```python
from build123d import *

# Parameters (mm, degrees)
EXTRUDE_1_DEPTH          = 6
PATTERN_CIRCULAR_1_COUNT = 20
SKETCH_2_R               = 2.55
CUT_EXTRUDE_1_DEPTH      = 19


with BuildPart() as part:
    # 스케치1 → 보스-돌출1 (new body)
    with BuildSketch(Plane(origin=(0, 0, 0), x_dir=(0, 0, -1), z_dir=(1, 0, 0))):
        with BuildLine():
            ThreePointArc((0, 12), (1.10558919, 10.60769458), (1.5, 8.874119675))
            ThreePointArc((1.5, 8.874119675), (0, -9), (-1.5, 8.874119675))
            ThreePointArc((-1.5, 8.874119675), (-1.10558919, 10.60769458), (0, 12))
        make_face()
    extrude_1 = extrude(amount=EXTRUDE_1_DEPTH)

    # 원형 패턴1: 보스-돌출1 ×20 about axis
    pattern_circular_1_axis = Axis((0, 0, 0), (1, 0, 0))
    for i in range(1, PATTERN_CIRCULAR_1_COUNT):
        add(extrude_1.rotate(pattern_circular_1_axis, i * 360 / PATTERN_CIRCULAR_1_COUNT))

    # 스케치2 → 컷-돌출1 (cut, through all)
    with BuildSketch(Plane(origin=(6, 0, 0), x_dir=(0, 0, -1), z_dir=(1, 0, 0))):
        Circle(SKETCH_2_R)
    extrude(amount=-CUT_EXTRUDE_1_DEPTH, mode=Mode.SUBTRACT)


solid = part.part
```
The listing builds one solid part. Answer for the finished solid, in the listing's coordinates (mm). Coordinates: 2 decimals unless noted, no trailing zeros. Write each loop counter-clockwise with the first axis right and the second up, starting at its lowest first coordinate (ties: lowest second). Pieces come first, ordered by that corner, then holes. Notation, with made-up numbers: M -35.75,25 L 6.25,25 A11 ccw 6.25,35 Z; hole C 34.25,-29.75 d8. An arc over 180 degrees is marked long. Use a Markdown table: item, result. Add a question column.
1. Straight lines are drawn through the part: line 1 along Z through (x, y) = (2.2, 10.75); line 2 along Y through (x, z) = (2.2, -1); line 3 along Y through (x, z) = (3.4, -9.75). For each, find the intervals that lie inside material, in ascending order. Write a range as [from, to].
2. Given P1, Ø10, axis at y = -5, z = -6, coming from the -X side; P2, Ø2, axis at x = 4, z = -6.5, coming from the +Y side; P3, Ø1.5, axis at x = 5, z = 5.5, coming from the +Y side; P4, Ø1.5, axis at x = 2.5, y = -0.5, coming from the -Z side, each flat-ended and moving along its own axis, determine where each tip first touches the part or whether it passes through.
3. For a pull along Y with two mould halves and no side action, classify faces 1 (the cylindrical face through (2.958, 5.518, 9.322)), 2 (the cylindrical face through (2.96, 7.16, -8.13)) as +Y half, -Y half, draft (parallel to the pull), parting line (faces both ways), or undercut.
4. Section B-B (y = -10) is taken. Give the vertices of the cut face in (x, z).
5. Section D-D (z = -6) is taken. Give the vertices of the cut face in (x, y).
6. Section A-A (z = -2) is taken. Give the vertices of the cut face in (x, y), plus the area to 3 significant figures.
7. Section C-C (z = 8) is taken. Give the vertices of the cut face in (x, y).
Data:
| question | item | result |
|---|---|---|
| 1 | line 1 | z = [-4.06, -2.57], [-1.03, 1.03], [2.57, 4.06] |
| 1 | line 2 | y = [-10.81, -2.35], [2.35, 10.81] |
| 1 | line 3 | y = [-4.33, -1.7], [-1.4, 1.4], [1.7, 4.33] |
| 2 | P1 | stops at x = 0 |
| 2 | P2 | stops at y = 9.71 |
| 2 | P3 | stops at y = 9.59 |
| 2 | P4 | stops at z = -12 |
| 3 | face 1 | undercut |
| 3 | face 2 | undercut |
| 4 | outline | M 0,-4.29 L 6,-4.29 L 6,-1.87 L 0,-1.87 Z; M 0,-1.34 L 6,-1.34 L 6,1.34 L 0,1.34 Z; M 0,1.87 L 6,1.87 L 6,4.29 L 0,4.29 Z |
| 5 | outline | M 0,-9.51 L 6,-9.51 L 6,9.51 L 0,9.51 Z |
| 6 | outline | M 0,-10.17 L 6,-10.17 L 6,-1.58 L 0,-1.58 Z; M 0,1.58 L 6,1.58 L 6,10.17 L 0,10.17 Z |
| 6 | area | 103 mm2 |
| 7 | outline | M 0,-7.14 L 6,-7.14 L 6,7.14 L 0,7.14 Z |
